Could you check a few things on this drawing? It's one solid part, dimensions in mm from its lowest x, y, z. A direction names the side the tool comes from. Round coordinates to 2 decimals unless told otherwise and drop trailing zeros. Write each loop counter-clockwise with the first axis right and the second up, starting at its lowest first coordinate (ties: lowest second). Pieces come first, ordered by that corner, then holes. Notation, with made-up numbers: (70, 8) -> (90, 8) arc R15 cw to (90, 22) -> close; hole circle Ø3 at (87, 75). An arc over 180 degrees is marked (long way). Put each result on its own line as item: value. Start each with the question number.
1) I want a section at A-A, the plane z = 0.7. List the corners of the cut face in (x, y) for me, then the cut area to 3 significant figures.
2) We'd pull the mould along Y, two halves only. Please class the marked faces 3, 4 and 5: released by +Y, released by -Y, zero draft, split by the parting line, or undercut.
3) Which directions (+Z, -Z, +X, -X, +Y, -Y) give clear straight access to the entire face, cutting with the end or side of a thin tool? Please do the marked faces 1 and 2.
4) I want a section at B-B, the plane x = 6.1. List the corners of the cut face in (y, z) for me, then the cut area to 3 significant figures.
5) I want a section at D-D, the plane x = 8.75. List the corners of the cut face in (y, z) for me, then the cut area to 3 significant figures.
6) I want a section at C-C, the plane y = 5.9. List the corners of the cut face in (x, z) for me, then the cut area to 3 significant figures.
7) If I drill on line 1 along Y through (x, z) = (6.1, 0.85); line 2 along X through (y, z) = (5.5, 1.7); line 3 along Z through (x, y) = (3.25, 6), over which ranges is the centre line in solid material (lowest first)? Write a range as [from, to].
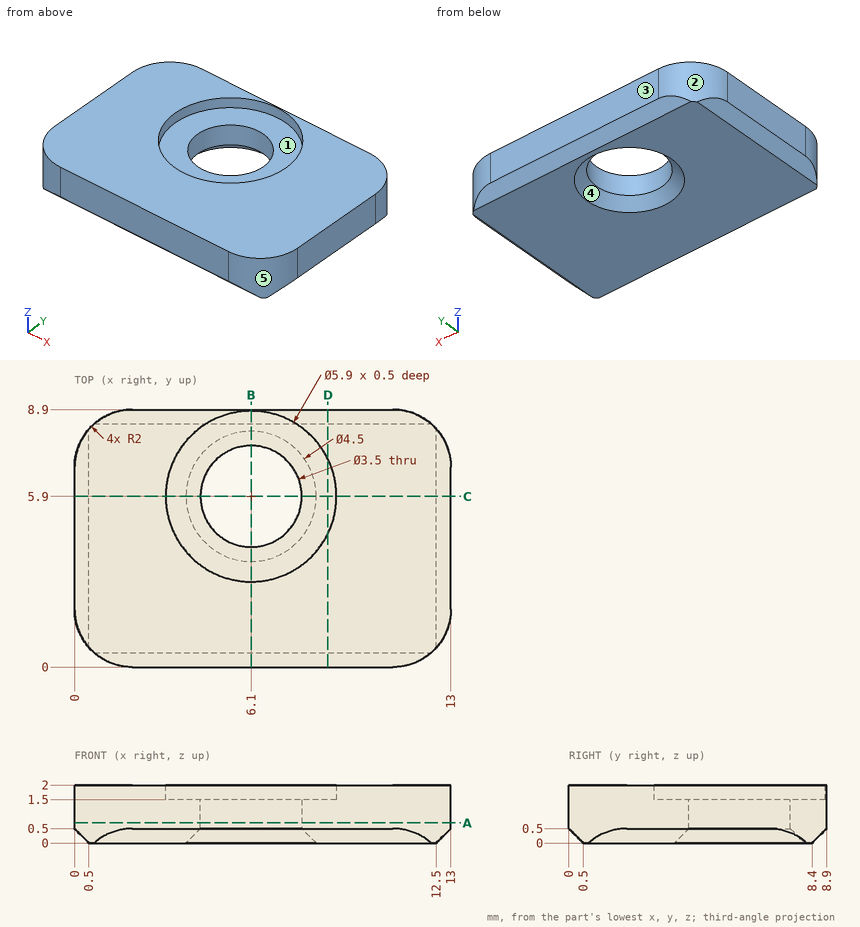
Findings:
1. outline: (0, 2) arc R2 ccw to (2, 0) -> (11, 0) arc R2 ccw to (13, 2) -> (13, 6.9) arc R2 ccw to (11, 8.9) -> (2, 8.9) arc R2 ccw to (0, 6.9) -> close; hole circle Ø3.5 at (6.1, 5.9)
1. area: 103 mm2
2. face 3: released by +Y
2. face 4: undercut
2. face 5: released by -Y
3. face 1: +Z
3. face 2: +Z, -Z, -X, +Y
4. outline: (0, 0.5) -> (0.5, 0) -> (3.65, 0) -> (4.15, 0.5) -> (4.15, 1.5) -> (2.95, 1.5) -> (2.95, 2) -> (0, 2) -> close; (7.65, 0.5) -> (8.15, 0) -> (8.4, 0) -> (8.9, 0.5) -> (8.9, 2) -> (8.85, 2) -> (8.85, 1.5) -> (7.65, 1.5) -> close
4. area: 9.10 mm2
5. outline: (0, 0.5) -> (0.5, 0) -> (8.4, 0) -> (8.9, 0.5) -> (8.9, 2) -> (7.2, 2) -> (7.2, 1.5) -> (4.6, 1.5) -> (4.6, 2) -> (0, 2) -> close
5. area: 16.3 mm2
6. outline: (0, 0.5) -> (0.5, 0) -> (3.85, 0) -> (4.35, 0.5) -> (4.35, 1.5) -> (3.15, 1.5) -> (3.15, 2) -> (0, 2) -> close; (7.85, 0.5) -> (8.35, 0) -> (12.5, 0) -> (13, 0.5) -> (13, 2) -> (9.05, 2) -> (9.05, 1.5) -> (7.85, 1.5) -> close
6. area: 17.3 mm2
7. line 1: y = [0, 4.15], [7.65, 8.9]
7. line 2: x = [0, 3.18], [9.02, 13]
7. line 3: z = [0, 1.5]
